from build123d import *

# Parameters (mm, degrees)
SKETCH1_W           = 1250
SKETCH1_H           = 600
SKETCH1_W_2         = 1220
SKETCH1_H_2         = 570
SKETCH1_H_3         = 5
BOSS_EXTRUDE1_DEPTH = 300
SKETCH2_W           = 1250
SKETCH2_H           = 600
BOSS_EXTRUDE2_DEPTH = 5


with BuildPart() as part:
    # Sketch1 → Boss-Extrude1 (new body)
    # profile 1 of 3: a face of its own
    with BuildSketch(Plane.XY):
        with Locations((0, -300)):
            Rectangle(SKETCH1_W, SKETCH1_H)
        with Locations((0, -300)):
            Rectangle(SKETCH1_W_2, SKETCH1_H_2, mode=Mode.SUBTRACT)
    # profile 2 of 3: a face of its own
    with BuildSketch(Plane.XY):
        with Locations((0, -302.5)):
            Rectangle(SKETCH1_W_2, SKETCH1_H_3)
    # profile 3 of 3: a face of its own
    with BuildSketch(Plane.XY):
        with Locations((0, -297.5)):
            Rectangle(SKETCH1_W_2, SKETCH1_H_3)
    extrude(amount=BOSS_EXTRUDE1_DEPTH)

    # Sketch2 → Boss-Extrude2 (add)
    with BuildSketch(Plane(origin=(0, 0, 0), x_dir=(-1, 0, 0), z_dir=(0, 0, -1))):
        with Locations((0, -300)):
            Rectangle(SKETCH2_W, SKETCH2_H)
    extrude(amount=-BOSS_EXTRUDE2_DEPTH)


solid = part.part
Can you work these out from the model? Positions are in its coordinate system, mm. A direction names the side the tool comes from. Give positions to 0.01 mm unless a question says otherwise; leave off trailing zeros. Order: outer loops, then holes, each group sorted by start corner. A loop starts at its lowest first (then second) coordinate and runs counter-clockwise, first axis right, second up. Notation, with made-up numbers: M 48.25,37.25 L 67.25,37.25 A23 cw 67.25,72.25 Z; hole C -13,46.25 d2. An arc over 180 degrees is marked long. Use one line per item in the form item = value.
Item 1: If we section it at B-B, the plane y = -218: Write out the boundary of the cut face in (x, z).
Values follow:
outline = M -625,0 L 625,0 L 625,300 L 610,300 L 610,5 L -610,5 L -610,300 L -625,300 Z
Item 2: If we section it at A-A, the plane z = 85.5: Write out the boundary of the cut face in (x, y), and give its area (3 significant figures).
Values follow:
outline = M -625,-600 L 625,-600 L 625,0 L -625,0 Z; hole M -610,-585 L 610,-585 L 610,-305 L -610,-305 Z; hole M -610,-295 L 610,-295 L 610,-15 L -610,-15 Z
area = 66,800 mm^2
Item 3: If I drill on line 1 along Y through (x, z) = (482, 112.5); line 2 along X through (y, z) = (-433.5, 75.5); line 3 along Z through (x, y) = (297.5, -387), over which ranges is the centre line in solid material (lowest first)? Write a range as [from, to].
Values follow:
line_1 = [-600, -585], [-305, -295], [-15, 0]
line_2 = [-625, -610], [610, 625]
line_3 = [0, 5]
Item 4: If we section it at C-C, the plane x = -274: Write out the boundary of the cut face in (y, z), and give its area (3 significant figures).
Values follow:
outline = M -600,0 L 0,0 L 0,300 L -15,300 L -15,5 L -295,5 L -295,300 L -305,300 L -305,5 L -585,5 L -585,300 L -600,300 Z
area = 14,800 mm^2
Item 5: For faces 1 (the flat face through (-9, -296, 0)), 2 (the flat face through (-9, -295, 150)), which set-ups out of +Z, -Z, +X, -X, +Y, -Y let a thin tool reach every point of the face, with its end or its side?
Values follow:
face_1 = -Z, +X, -X, +Y, -Y
face_2 = +Z
Item 6: Thinking about a two-plate mould opening in X: for faces 3 (the flat face through (-3, -299, 300)), 4 (the flat face through (-610, -157, 150)), 5 (the flat face through (625, -304, 148)), which applies, pulls with the +X half, pulls with the -X half, needs draft (parallel to the pull), parting line crosses it, or undercut?
Values follow:
face_3 = needs draft
face_4 = undercut
face_5 = pulls with the +X half
Item 7: Will this pin go through, and if not, where does the flat tip stop? pin 1 Ø1 at (x, y) = (490.5, -176.5) entering from +Z.
Values follow:
pin_1 = 5
